```python
from build123d import *

# Parameters (mm, degrees)
SKETCH_W     = 26
SKETCH_H     = 56
SKETCH_R     = 3
SKETCH_R_2   = 12
PAD_DEPTH    = 1
PAD001_DEPTH = 3


with BuildPart() as part:
    # Sketch → Pad (new body)
    with BuildSketch(Plane.XY):
        Rectangle(SKETCH_W, SKETCH_H)
        with Locations((0, 20.6375)):
            Circle(SKETCH_R, mode=Mode.SUBTRACT)
        with Locations((0, -20.6375)):
            Circle(SKETCH_R, mode=Mode.SUBTRACT)
        Circle(SKETCH_R_2, mode=Mode.SUBTRACT)
    extrude(amount=PAD_DEPTH)

    # Sketch001 → Pad001 (join)
    with BuildSketch(Plane.XY):
        with BuildLine():
            ThreePointArc((-3, 28), (-9.550145, 24.550145), (-13, 18))
            Line((-13, 18), (-13, 28))
            Line((-13, 28), (-3, 28))
        make_face()
        with BuildLine():
            ThreePointArc((13, 18), (9.550145, 24.550145), (3, 28))
            Line((13, 28), (3, 28))
            Line((13, 18), (13, 28))
        make_face()
        with BuildLine():
            ThreePointArc((-13, -18), (-9.550145, -24.550145), (-3, -28))
            Line((-13, -28), (-3, -28))
            Line((-13, -18), (-13, -28))
        make_face()
        with BuildLine():
            ThreePointArc((3, -28), (9.550145, -24.550145), (13, -18))
            Line((13, -28), (13, -18))
            Line((3, -28), (13, -28))
        make_face()
    extrude(amount=PAD001_DEPTH)


solid = part.part
```
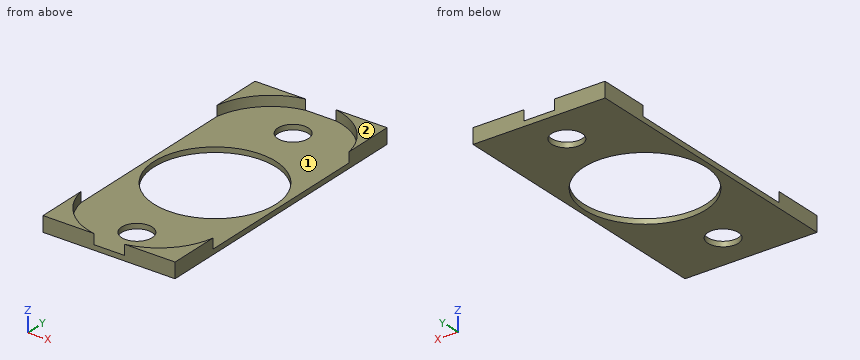
Could you check a few things on this model? Use its own coordinates, in mm. Face numbers are marked on the shaded views. Coordinates: 2 decimals unless noted, no trailing zeros. Write each loop counter-clockwise with the first axis right and the second up, starting at its lowest first coordinate (ties: lowest second). Pieces come first, ordered by that corner, then holes. Notation, with made-up numbers: M -25,86.25 L 20,86.25 A25 cw 20,124.25 Z; hole C 11,-21 d7. An arc over 180 degrees is marked long. Answer as CSV lines item,"result". Start each with the question number.
1) Please list where these lines run through material, in increasing order: line 1 (Y direction, x = 0, z = 0.4); line 2 (Y direction, x = 1.75, z = 0.45); line 3 (X direction, y = -21, z = 2.6). Write a range as from..to.
2) I want a section at D-D, the plane x = -11.25. Please give me the cut outline in (y, z), and give its area (3 significant figures).
3) I want a section at C-C, the plane z = 2.3. Please give me the cut outline in (x, y).
4) I want a section at A-A, the plane x = 0. Please give me the cut outline in (y, z).
5) We'd pull the mould along Y, two halves only. Please class the marked faces 1 and 2: +Y half, -Y half, draft (parallel to the pull), parting line (faces both ways), or undercut.
6) For P1, Ø4, axis at x = 9, y = 17.5, coming from the +Z side, with a flat end and sliding along its axis, tell me the tip position at first contact or that it passes through.
7) I want a section at B-B, the plane y = 0. Please give me the cut outline in (x, z), and give its area (3 significant figures).
Data:
1,line 1,"y = -28..-23.64, -17.64..-12, 12..17.64, 23.64..28"
1,line 2,"y = -28..-23.07, -18.2..-11.87, 11.87..18.2, 23.07..28"
1,line 3,"x = -13..-12.04, 12.04..13"
2,outline,"M -28,0 L -4.18,0 L -4.18,1 L -22.43,1 L -22.43,3 L -28,3 Z; M 4.18,0 L 28,0 L 28,3 L 22.43,3 L 22.43,1 L 4.18,1 Z"
2,area,"69.9 mm^2"
3,outline,"M -13,-28 L -3,-28 A12.5 cw -13,-18 Z; M -13,18 A12.5 cw -3,28 L -13,28 Z; M 3,-28 L 13,-28 L 13,-18 A12.5 cw Z; M 3,28 A12.5 cw 13,18 L 13,28 Z"
4,outline,"M -28,0 L -23.64,0 L -23.64,1 L -28,1 Z; M -17.64,0 L -12,0 L -12,1 L -17.64,1 Z; M 12,0 L 17.64,0 L 17.64,1 L 12,1 Z; M 23.64,0 L 28,0 L 28,1 L 23.64,1 Z"
5,face 1,"undercut"
5,face 2,"draft"
6,P1,"stops at z = 1"
7,outline,"M -13,0 L -12,0 L -12,1 L -13,1 Z; M 12,0 L 13,0 L 13,1 L 12,1 Z"
7,area,"2.00 mm^2"
